```python
from build123d import *

# Parameters (mm, degrees)
F0_R     = 10.9601
F0_R_2   = 12.7
F1_DEPTH = 25.4


with BuildPart() as f1:
    # F0 (on Top) → F1 (new body)
    with BuildSketch(Plane.XY):
        with BuildLine():
            ThreePointArc((5.08, 19.525683), (11.038189, 27.93156), (12.7, 38.1))
            ThreePointArc((12.7, 38.1), (0, 50.8), (-12.7, 38.1))
            ThreePointArc((-12.7, 38.1), (-11.038189, 27.93156), (-5.08, 19.525683))
            ThreePointArc((-5.08, 19.525683), (-9.703888, 13.905597), (-12.327043, 7.117022))
            ThreePointArc((-12.327043, 7.117022), (-16.894544, 1.451015), (-19.449737, -5.363432))
            ThreePointArc((-19.449737, -5.363432), (-29.708535, -4.406428), (-39.345568, -8.051477))
            ThreePointArc((-39.345568, -8.051477), (-43.994091, -25.4), (-26.645568, -30.048523))
            ThreePointArc((-26.645568, -30.048523), (-18.670346, -23.525132), (-14.369737, -14.16225))
            ThreePointArc((-14.369737, -14.16225), (-7.190656, -15.356612), (0, -14.234043))
            ThreePointArc((0, -14.234043), (7.190656, -15.356612), (14.369737, -14.16225))
            ThreePointArc((14.369737, -14.16225), (18.670346, -23.525132), (26.645568, -30.048523))
            ThreePointArc((26.645568, -30.048523), (43.994091, -25.4), (39.345568, -8.051477))
            ThreePointArc((39.345568, -8.051477), (29.708535, -4.406428), (19.449737, -5.363432))
            ThreePointArc((19.449737, -5.363432), (16.894544, 1.451015), (12.327043, 7.117022))
            ThreePointArc((12.327043, 7.117022), (9.703888, 13.905597), (5.08, 19.525683))
        make_face()
        with Locations((-32.995568, -19.05)):
            Circle(F0_R, mode=Mode.SUBTRACT)
        with Locations((32.995568, -19.05)):
            Circle(F0_R, mode=Mode.SUBTRACT)
        Circle(F0_R_2, mode=Mode.SUBTRACT)
        with Locations((0, 38.1)):
            Circle(F0_R, mode=Mode.SUBTRACT)
        Circle(F0_R_2)
        Circle(F0_R, mode=Mode.SUBTRACT)
    extrude(amount=F1_DEPTH)


solid = f1.part
```
Model file for the job. Use its own axes, mm. A direction names the side the tool comes from. Coordinates: 2 decimals unless noted, no trailing zeros. Write each loop counter-clockwise with the first axis right and the second up, starting at its lowest first coordinate (ties: lowest second). Pieces come first, ordered by that corner, then holes. Notation, with made-up numbers: (-25, -31.75) - (-2, -31.75) arc R30 cw to (-2, -5.75) - close; hole circle Ø1 at (-5, 25). An arc over 180 degrees is marked (long way). One line per item, written item: value. Start each with the question number.
1. Slice it at D-D (z = 6.5). Write the cut outline in (x, y).
2. Flat gauge pins, fed straight in: pin 1 (25 mm diameter, centred on x = 0, y = 0, fed in from -Z); pin 2 (5 mm diameter, centred on x = -32.5, z = 9, fed in from +Y); pin 3 (5 mm diameter, centred on y = 25, z = 13, fed in from -X); pin 4 (13 mm diameter, centred on x = 0, y = 38.1, fed in from +Z). Where does each tip first touch, or does it go through?
3. Probe line 1 (X direction, y = -28, z = 18.25); line 2 (X direction, y = -21.5, z = 23.25); line 3 (Y direction, x = 0, z = 15). List the from-to ranges inside material, lowest first. Write a range as from..to.
4. Slice it at C-C (x = 31.5). Write the cut outline in (y, z).
5. Mould opens along X. For faces 3 (the flat face through (-7, -9, 0)), 4 (the cylindrical face through (43.12, -23.25, 12.52)), 5 (the cylindrical face through (0.279, 50.797, 12.522)) say: released by +X, released by -X, zero draft, split by the parting line, or undercut.
6. Slice it at B-B (y = 43). Write the cut outline in (x, z).
7. Tool access for faces 1 (the flat face through (-7, -9, 25.4)), 2 (the cylindrical face through (18.58, -23.41, 12.52)): list every direction of +Z, -Z, +X, -X, +Y, -Y with a clear straight run to the whole face (end or side of a thin tool).
8. Slice it at A-A (y = -19.05). Write the cut outline in (x, z).
Answers below:
1. outline: (-39.35, -8.05) arc R12.7 ccw to (-26.65, -30.05) arc R22.86 ccw to (-14.37, -14.16) arc R22.86 ccw to (0, -14.23) arc R22.86 ccw to (14.37, -14.16) arc R22.86 ccw to (26.65, -30.05) arc R12.7 ccw to (39.35, -8.05) arc R22.86 ccw to (19.45, -5.36) arc R22.86 ccw to (12.33, 7.12) arc R22.86 ccw to (5.08, 19.53) arc R22.86 ccw to (12.7, 38.1) arc R12.7 ccw to (-12.7, 38.1) arc R22.86 ccw to (-5.08, 19.53) arc R22.86 ccw to (-12.33, 7.12) arc R22.86 ccw to (-19.45, -5.36) arc R22.86 ccw to start; hole circle Ø21.92 at (-33, -19.05); hole circle Ø21.92 at (0, 0); hole circle Ø21.92 at (0, 38.1); hole circle Ø21.92 at (33, -19.05)
2. pin 1: stops at z = 0
2. pin 2: stops at y = -4.45
2. pin 3: stops at x = -10.86
2. pin 4: passes through
3. line 1: x = -42.01..-39.32, -26.67..-23.27, 23.27..26.67, 39.32..42.01
3. line 2: x = -45.46..-43.68, -22.31..-17.27, 17.27..22.31, 43.68..45.46
3. line 3: y = -14.23..-10.96, 10.96..27.14, 49.06..50.8
4. outline: (-31.66, 0) - (-29.91, 0) - (-29.91, 25.4) - (-31.66, 25.4) - close; (-8.19, 0) - (-4.72, 0) - (-4.72, 25.4) - (-8.19, 25.4) - close
5. face 3: zero draft
5. face 4: undercut
5. face 5: split by the parting line
6. outline: (-11.72, 0) - (-9.8, 0) - (-9.8, 25.4) - (-11.72, 25.4) - close; (9.8, 0) - (11.72, 0) - (11.72, 25.4) - (9.8, 25.4) - close
7. face 1: +Z, +X, -X, +Y, -Y
7. face 2: +Z, -Z, -Y
8. outline: (-45.7, 0) - (-43.96, 0) - (-43.96, 25.4) - (-45.7, 25.4) - close; (-22.04, 0) - (-15.97, 0) - (-15.97, 25.4) - (-22.04, 25.4) - close; (15.97, 0) - (22.04, 0) - (22.04, 25.4) - (15.97, 25.4) - close; (43.96, 0) - (45.7, 0) - (45.7, 25.4) - (43.96, 25.4) - close
